from build123d import *

# Parameters (mm, degrees)
SKETCH2_W           = 8.0391
SKETCH2_H           = 4.1783
SKETCH2_W_2         = 15.0876
SKETCH2_H_2         = 5.588
SKETCH2_R           = 2.96545
BOSS_EXTRUDE1_DEPTH = 1.8034


with BuildPart() as part:
    # Sketch2 → Boss-Extrude1 (new body)
    with BuildSketch(Plane(origin=(0, 0, 0), x_dir=(0, 0, -1), z_dir=(1, 0, 0))):
        Polygon((6.35, 24.0792), (0, 24.0792), (0, 21.2344), (-1.8034, 21.2344), (-1.8034, 16.1544), (0, 16.1544), (0, 9.8044), (-1.8034, 9.8044), (-1.8034, 4.7244), (6.35, 4.7244), (6.35, 1.5494), (46.863, 1.5494), (46.863, 4.7244), (84.963, 4.7244), (84.963, 12.0396), (86.7664, 12.0396), (86.7664, 4.7244), (89.3064, 4.7244), (89.3064, 24.0792), (53.213, 24.0792), (53.213, 27.2542), (6.35, 27.2542), align=None)
        with Locations((10.64895, 7.29615)):
            Rectangle(SKETCH2_W, SKETCH2_H, mode=Mode.SUBTRACT)
        with Locations((31.8008, 9.7155)):
            Rectangle(SKETCH2_W_2, SKETCH2_H_2, mode=Mode.SUBTRACT)
        with Locations((53.48605, 9.17575)):
            Circle(SKETCH2_R, mode=Mode.SUBTRACT)
    extrude(amount=BOSS_EXTRUDE1_DEPTH)


solid = part.part
Input: part model. Units: mm. Frame: model coordinates. A direction names the side the tool comes from. Give positions to 0.01 mm unless a question says otherwise; leave off trailing zeros. Order: outer loops, then holes, each group sorted by start corner. A loop starts at its lowest first (then second) coordinate and runs counter-clockwise, first axis right, second up. Notation, with made-up numbers: M 73.5,43 L 103.5,43 A22 ccw 103.5,72 Z; hole C 82.5,62.5 d7. An arc over 180 degrees is marked long. Answer as a JSON object with one key per item and string values.
1. Cut plane D-D, the plane y = 22.75. Output: boundary loops of the cut face in (x, z), and give its area (3 significant figures).
Result sheet:
{"outline": "M 0,-89.31 L 1.8,-89.31 L 1.8,0 L 0,0 Z", "area": "161 mm²"}
2. First-contact query: P1, Ø0.9, axis at x = 1, z = -88, coming from the -Y side; P2, Ø0.5, axis at x = 1, z = -86, coming from the -Y side; P3, Ø0.9, axis at x = 1, y = 10.5, coming from the +Z side. Flat tips, straight axial feed; report the tip coordinate or a pass-through.
Result sheet:
{"P1": "y = 4.72", "P2": "y = 12.04", "P3": "z = 0"}
3. Reachability of faces 4 (the flat face through (1, 3, -46.863)), 5 (the flat face through (1, 8, -86.766)), 6 (the flat face through (1, 21.234, 1)) from +Z, -Z, +X, -X, +Y, -Y: full face, straight path, thin tool, end or side. Return the list, or none.
Result sheet:
{"face 4": "-Z, +X, -X, -Y", "face 5": "+X, -X, -Y", "face 6": "+Z, +X, -X, +Y"}
4. Cut plane A-A, the plane y = 7.75. Output: boundary loops of the cut face in (x, z).
Result sheet:
{"outline": "M 0,-89.31 L 1.8,-89.31 L 1.8,-86.77 L 0,-86.77 Z; M 0,-84.96 L 1.8,-84.96 L 1.8,-56.09 L 0,-56.09 Z; M 0,-50.89 L 1.8,-50.89 L 1.8,-39.34 L 0,-39.34 Z; M 0,-24.26 L 1.8,-24.26 L 1.8,-14.67 L 0,-14.67 Z; M 0,-6.63 L 1.8,-6.63 L 1.8,1.8 L 0,1.8 Z"}
5. Ray query, line 1 (Y direction, x = 0.9, z = -30.5); line 2 (Y direction, x = 0.65, z = -1.5); line 3 (Z direction, x = 0.2, y = 14). Return the intervals inside material, ascending. Write a range as [from, to].
Result sheet:
{"line 1": "[1.55, 6.92], [12.51, 27.25]", "line 2": "[4.72, 24.08]", "line 3": "[-89.31, 0]"}
6. Cut plane C-C, the plane x = 1.25. State how many separate pieces and enclosed holes the cut face has, and give its area (3 significant figures).
Result sheet:
{"separate pieces": "1", "enclosed holes": "3", "area": "1,870 mm²"}
7. Cut plane B-B, the plane z = -55. Output: boundary loops of the cut face in (x, y).
Result sheet:
{"outline": "M 0,4.72 L 1.8,4.72 L 1.8,6.63 L 0,6.63 Z; M 0,11.73 L 1.8,11.73 L 1.8,24.08 L 0,24.08 Z"}
8. Pull-direction query (Z, two-part tool) for faces 1 (the flat face through (1, 4.724, -2)), 2 (the flat face through (1, 7, -14.668)), 3 (the flat face through (1, 23, 0)); classes: +Z half, -Z half, draft (parallel to the pull), parting line (faces both ways), or undercut.
Result sheet:
{"face 1": "draft", "face 2": "undercut", "face 3": "+Z half"}
